Build history of the part. All positions in model axes, mm. A direction names the side the tool comes from. Give positions to 0.01 mm unless a question says otherwise; leave off trailing zeros. Write each loop counter-clockwise with the first axis right and the second up, starting at its lowest first coordinate (ties: lowest second). Pieces come first, ordered by that corner, then holes.
from build123d import *

# Parameters (mm, degrees)
F1_DEPTH  = 80
F2_R      = 2.5
F3_DEPTH  = 10
F2_W      = 56
F2_H      = 32
F2_W_2    = 52
F2_H_2    = 28
F4_DEPTH  = 20
F6_W      = 56
F6_H      = 32
F6_W_2    = 45
F6_H_2    = 26
F7_DEPTH  = 2
F8_R      = 1.5
F9_R      = 3
F10_DEPTH = 10


with BuildPart() as f1:
    # F0 (on Right) → F1 (new body)
    with BuildSketch(Plane.YZ):
        Polygon((0, 32), (0, 0), (24, 0), (24, 5), (22, 5), (22, 2), (2, 2), (2, 22), (5, 22), (5, 32), align=None)
    extrude(amount=F1_DEPTH)

    # F2 (on Front) → F3 (cut)
    with BuildSketch(Plane.XZ):
        with Locations((5, 12)):
            Circle(F2_R)
        with Locations((75, 12)):
            Circle(F2_R)
    extrude(amount=-F3_DEPTH, mode=Mode.SUBTRACT)

    # F2 (on Front) → F4 (join)
    with BuildSketch(Plane.XZ):
        with Locations((40, 16)):
            Rectangle(F2_W, F2_H)
        with Locations((40, 16)):
            Rectangle(F2_W_2, F2_H_2, mode=Mode.SUBTRACT)
    extrude(amount=F4_DEPTH)

    # F6 (on offset) → F7 (join)
    with BuildSketch(Plane.XZ.offset(20)):
        with Locations((40, 16)):
            Rectangle(F6_W, F6_H)
        with Locations((40, 16)):
            Rectangle(F6_W_2, F6_H_2, mode=Mode.SUBTRACT)
    extrude(amount=F7_DEPTH)

    # F8
    f8_edges = [f1.edges().sort_by_distance(p)[0] for p in [
        (68, -22, 16),
        (40, -22, 32),
        (12, -22, 16),
        (40, -22, 0),
        (68, -11, 32),
        (12, -11, 32),
        (12, -11, 0),
        (68, -11, 0),
        (40, 22, 5),
        (40, 5, 32),
        (6, 0, 32),
        (74, 0, 32),
        (6, 0, 0),
        (74, 0, 0),
    ]]
    fillet(f8_edges, radius=F8_R)

    # F9 (on Top) → F10 (cut)
    with BuildSketch(Plane.XY):
        with Locations((20, -5.453821)):
            Circle(F9_R)
    extrude(amount=F10_DEPTH, mode=Mode.SUBTRACT)


solid = f1.part
1. Saw through at B-B on z = 12. Give the cut face in (x, y).
2. Drop flat-ended pins along their axis: pin 1 (5 mm diameter, centred on y = -3.5, z = 18.5, fed in from +X); pin 2 (6 mm diameter, centred on x = 5, z = 12, fed in from +Y); pin 3 (0.6 mm diameter, centred on x = 36, y = -21.5, fed in from -Z). Give the stop position or say it passes through.
3. Saw through at D-D on z = 26.5. Give the cut face in (x, y), plus the area to 3 significant figures.
4. Saw through at C-C on y = -15. Give the cut face in (x, z), plus the area to 3 significant figures.
5. Drill centre lines: line 1 along Y through (x, z) = (56, 2.5); line 2 along X through (y, z) = (-12.5, 23); line 3 along Y through (x, z) = (16, 14). Where is each one in solid material? Low to high.
6. Saw through at A-A on x = 5. Give the cut face in (y, z).
7. 3-axis set-ups, long thin cutter, end or side, ignore diameter. For faces 1 (the face through (39, 5, 26)), 2 (the face through (67.57, -9.35, 31.55)), 3 (the face through (62.5, -21, 16)), 4 (the face through (39, 3, 22)), 5 (the face through (12.43, -9.65, 0.45)): which of +Z, -Z, +X, -X, +Y, -Y reach the whole face in a straight line?
8. Mould opens along X. For faces 6 (the face through (12.43, -9.35, 31.55)), 7 (the face through (40, -22, 30)), 8 (the face through (40, -10, 30)) say: pulls with the +X half, pulls with the -X half, needs draft (parallel to the pull), parting line crosses it, or undercut.
Outcome:
1. outline: (0, 0) - (2.5, 0) - (2.5, 2) - (0, 2) - close; (7.5, 0) - (12, 0) - (12, -20.5) arc R1.5 ccw to (13.5, -22) - (17.5, -22) - (17.5, -20) - (14, -20) - (14, 0) - (66, 0) - (66, -20) - (62.5, -20) - (62.5, -22) - (66.5, -22) arc R1.5 ccw to (68, -20.5) - (68, 0) - (72.5, 0) - (72.5, 2) - (7.5, 2) - close; (77.5, 0) - (80, 0) - (80, 2) - (77.5, 2) - close
2. pin 1: stops at x = 68
2. pin 2: stops at y = 2
2. pin 3: stops at z = 0.17
3. outline: (0, 0) - (12, 0) - (12, -20.5) arc R1.5 ccw to (13.5, -22) - (17.5, -22) - (17.5, -20) - (14, -20) - (14, 0) - (66, 0) - (66, -20) - (62.5, -20) - (62.5, -22) - (66.5, -22) arc R1.5 ccw to (68, -20.5) - (68, 0) - (80, 0) - (80, 5) - (0, 5) - close
3. area: 501 mm2
4. outline: (12, 1.5) arc R1.5 ccw to (13.5, 0) - (66.5, 0) arc R1.5 ccw to (68, 1.5) - (68, 30.5) arc R1.5 ccw to (66.5, 32) - (13.5, 32) arc R1.5 ccw to (12, 30.5) - close; hole (14, 2) - (66, 2) - (66, 30) - (14, 30) - close
4. area: 334 mm2
5. line 1: y = -22 to -20, 0 to 2, 22 to 24
5. line 2: x = 12 to 14, 66 to 68
5. line 3: y = -22 to -20, 0 to 2
6. outline: (0, 1.5) arc R1.5 ccw to (1.5, 0) - (24, 0) - (24, 5) - (23.5, 5) arc R1.5 ccw to (22, 3.5) - (22, 2) - (2, 2) - (2, 9.5) - (0, 9.5) - close; (0, 14.5) - (2, 14.5) - (2, 22) - (5, 22) - (5, 30.5) arc R1.5 ccw to (3.5, 32) - (1.5, 32) arc R1.5 ccw to (0, 30.5) - close
7. face 1: +Z, +X, -X, +Y
7. face 2: +Z, +X, -Y
7. face 3: -Y
7. face 4: +X, -X, +Y
7. face 5: -Z, -X, -Y
8. face 6: pulls with the -X half
8. face 7: needs draft
8. face 8: undercut
